Could you check a few things on this drawing? It's one solid part, dimensions in mm from its lowest x, y, z. A direction names the side the tool comes from. Give positions to 0.01 mm unless a question says otherwise; leave off trailing zeros. Loops run counter-clockwise (first coordinate to the right, second up) from the corner with the lowest first, then second, coordinate; pieces in that order, holes last. Notation, with made-up numbers: (-27, 53) - (26, 53) arc R23 ccw to (26, 86) - close; hole circle Ø10 at (-25.75, -4.75). An arc over 180 degrees is marked (long way). Use a Markdown table: item, result.
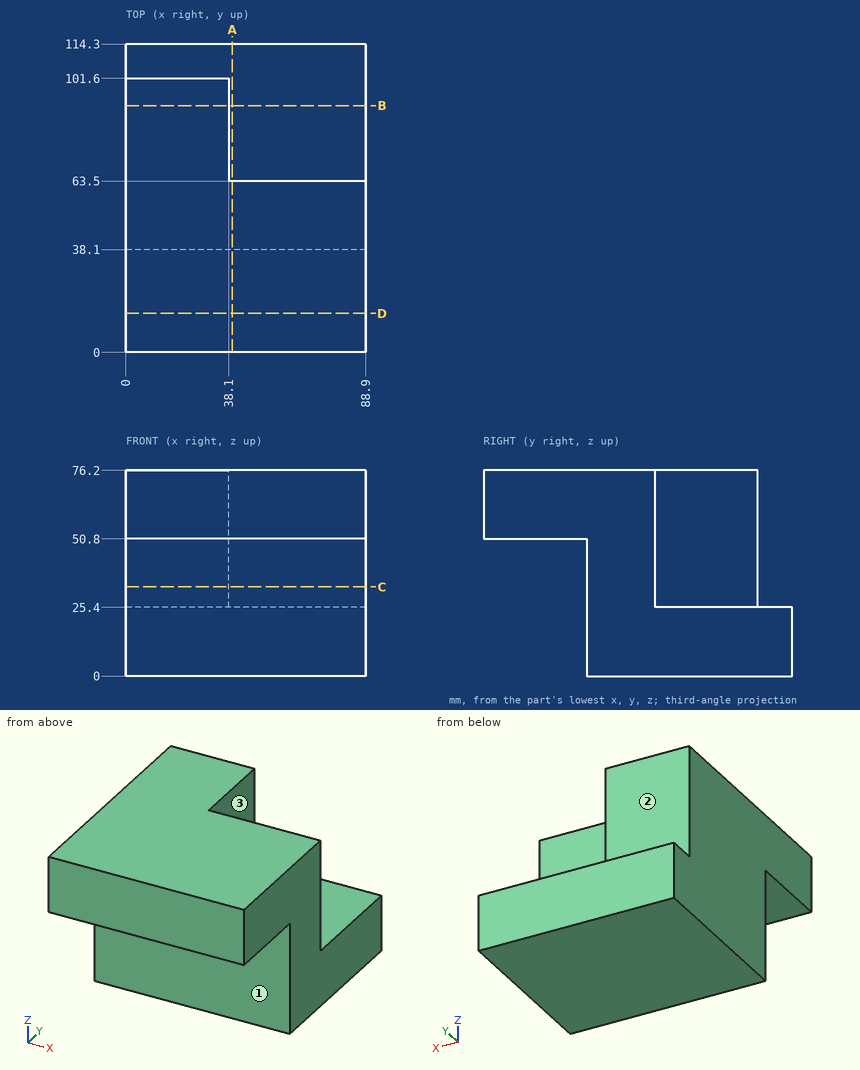
(1) Suppose I cut it at C-C on z = 33. Write out the boundary of the cut face in (x, y).
A:
| item | result |
|---|---|
| outline | (0, 38.1) - (88.9, 38.1) - (88.9, 63.5) - (38.1, 63.5) - (38.1, 101.6) - (0, 101.6) - close |
(2) Suppose I cut it at A-A on x = 39.5. Write out the boundary of the cut face in (y, z).
A:
| item | result |
|---|---|
| outline | (0, 50.8) - (38.1, 50.8) - (38.1, 0) - (114.3, 0) - (114.3, 25.4) - (63.5, 25.4) - (63.5, 76.2) - (0, 76.2) - close |
(3) Suppose I cut it at D-D on y = 14.5. Write out the boundary of the cut face in (x, z), plus the area to 3 significant figures.
A:
| item | result |
|---|---|
| outline | (0, 50.8) - (88.9, 50.8) - (88.9, 76.2) - (0, 76.2) - close |
| area | 2,260 mm2 |
(4) On a 3-axis mill with a long thin cutter (end or side, diameter ignored), from which of +Z, -Z, +X, -X, +Y, -Y can I reach the whole of each face in a straight line? I mean the marked faces 1, 2 and 3. Say none if no direction works.
A:
| item | result |
|---|---|
| face 1 | -Z, +X, -X, -Y |
| face 2 | +Z, +X, -X, +Y |
| face 3 | +Z, +X, +Y |
(5) If I drill on line 1 (Z direction, x = 50, y = 20.5); line 2 (Y direction, x = 54.5, z = 62.5); line 3 (X direction, y = 85, z = 59.5), over which ranges is the centre line in solid material (lowest first)?
A:
| item | result |
|---|---|
| line 1 | 50.8 to 76.2 |
| line 2 | 0 to 63.5 |
| line 3 | 0 to 38.1 |
(6) Suppose I cut it at B-B on y = 91.5. Write out the boundary of the cut face in (x, z), plus the area to 3 significant figures.
A:
| item | result |
|---|---|
| outline | (0, 0) - (88.9, 0) - (88.9, 25.4) - (38.1, 25.4) - (38.1, 76.2) - (0, 76.2) - close |
| area | 4,190 mm2 |
(7) Will these pins go through, and if not, where does the flat tip stop? pin 1 (5 mm diameter, centred on x = 31.5, z = 10, fed in from -Y); pin 2 (6 mm diameter, centred on x = 30, z = 39, fed in from +Y); pin 3 (12 mm diameter, centred on x = 48, y = 11.5, fed in from -Z).
A:
| item | result |
|---|---|
| pin 1 | y = 38.1 |
| pin 2 | y = 101.6 |
| pin 3 | z = 50.8 |
